Geometry check sheet. Reference: the model listing, model coordinates, mm. A direction names the side the tool comes from. Coordinates: 2 decimals unless noted, no trailing zeros. Write each loop counter-clockwise with the first axis right and the second up, starting at its lowest first coordinate (ties: lowest second). Pieces come first, ordered by that corner, then holes. Notation, with made-up numbers: (34.25, 33.5) -> (44.25, 33.5) arc R14 cw to (44.25, 57.5) -> close; hole circle Ø4 at (7, 25). An arc over 180 degrees is marked (long way). Put each result on its own line as item: value. Start each with the question number.
Autodesk Inventor part; units mm, degrees
ref_plane "YZ Plane" through (0, 0, 0) normal (1, 0, 0) x (0, 1, 0)
ref_plane "XZ Plane" through (0, 0, 0) normal (0, 1, 0) x (-1, 0, 0)
ref_plane "XY Plane" through (0, 0, 0) normal (0, 0, 1) x (1, 0, 0)
sketch "Sketch1" plane through (0, 0, 0) normal (0, 0, 1) x (1, 0, 0)
  line L0 (0, 0) -> (34, 0)
  line L1 (34, 0) -> (34, 69.8)
  line L2 (34, 69.8) -> (0, 69.8)
  line L3 (0, 69.8) -> (0, 0)
  line L4 (34, 69.8) -> (0, 69.8)
  line L5 (0, 69.8) -> (0, 0)
  line L6 (0, 0) -> (34, 0)
  line L7 (34, 0) -> (34, 69.8)
  dimension "d4" = 34
  dimension "d5" = 69.8
extrude "Extrusion1" add sketch "Sketch1" along normal blind 3.8
sketch "Sketch3" plane through (0, 0, 3.8) normal (0, 0, 1) x (1, 0, 0)
  line L0 (34, 69.8) -> (0, 69.8)
  line L1 (0, 0) -> (34, 0)
  line L2 (30, 69.8) -> (4, 69.8)
  line L3 (4, 69.8) -> (4, 0)
  line L4 (4, 0) -> (30, 0)
  line L5 (30, 0) -> (30, 69.8)
  line L6 (0, 69.8) -> (0, 0)
  line L7 (34, 0) -> (34, 69.8)
  dimension "d6" = 26
  dimension "d7" = 4
  dimension "d8" = 4
extrude "Extrusion3" add sketch "Sketch3" along normal blind 2.4 contours L5 L1 L3 L0
sketch "Sketch4" plane through (0, 0, 6.2) normal (0, 0, 1) x (1, 0, 0)
  point P0 (0, 0)
sketch "Sketch5" plane through (0, 0, 6.2) normal (0, 0, 1) x (1, 0, 0)
  line L0 (30, 69.8) -> (4, 69.8)
  line L1 (23.4, 69.8) -> (11.4, 69.8)
  line L2 (11.4, 69.8) -> (11.4, 61)
  line L3 (11.4, 61) -> (23.4, 61)
  line L4 (23.4, 61) -> (23.4, 69.8)
  point P0 (0, 0)
  dimension "d11" = 12
extrude "Extrusion4" cut sketch "Sketch5" against normal blind 8
fillet "Fillet1" radius 2 1 edges at (17, 0, 6.2)
fillet "Fillet2" radius 5 2 edges at (11.4, 65.4, 6.2) (23.4, 65.4, 6.2)
chamfer "Chamfer1" distance 2 angle 45 1 edges at (17.4, 61, 6.2)
sketch "Sketch6" plane through (0, 0, 0) normal (0, 0, -1) x (-1, 0, 0)
  line L0 (-30, 2) -> (-4, 2)
  line L1 (-30, 2) -> (-30, 69.8)
  line L2 (-4, 2) -> (-30, 2)
  line L3 (-30, 2) -> (-30, 67)
  line L4 (-30, 67) -> (-4, 67)
  line L5 (-4, 67) -> (-4, 2)
  point P0 (0, 0)
extrude "Extrusion5" cut sketch "Sketch6" against normal blind 2
properties part number "battery_cover"
Item 1: Section check D-D, the plane x = 2. Enter the section's corners in (y, z), and give its area (3 significant figures).
Item 2: Go/stop test with flat-tipped pins: P1, Ø1.9, axis at y = 36.5, z = 5, coming from the +X side; P2, Ø10, axis at x = 21.5, y = 55.5, coming from the -Z side; P3, Ø0.6, axis at x = 12, z = 0.5, coming from the +Y side. Record where each tip stops, or that it passes through.
Item 3: Section check C-C, the plane x = 26.5. Enter the section's corners in (y, z), and give its area (3 significant figures).
Item 4: Mould release check, pull along X, two halves, no side actions. Record for faces 1 (the flat face through (34, 34, 2)), 2 (the flat face through (0, 35, 2)), 3 (the flat face through (17.6, 60, 5.2)), 4 (the cylindrical face through (9.313, 65.524, 5.264)): released by +X, released by -X, zero draft, split by the parting line, or undercut.
Item 5: Section check B-B, the plane x = 12.5. Enter the section's corners in (y, z), and give its area (3 significant figures).
Item 6: Access from +Z, -Z, +X, -X, +Y, -Y to the whole of each face (thin tool, end or side, straight path). Record for faces 5 (the flat face through (4, 35, 5)), 6 (the flat face through (27, 67, 1)), 7 (the flat face through (32, 35, 3.8)), 8 (the cylindrical face through (25.487, 65.676, 5.264)).
Item 7: Scan lines: line 1 along Y through (x, z) = (28.5, 0.5); line 2 along Y through (x, z) = (14.5, 3); line 3 along Z through (x, y) = (21.5, 48). Record each from-to range of solid material in increasing order. Write a range as [from, to].
Item 8: Section check A-A, the plane y = 30.5. Enter the section's corners in (x, z), and give its area (3 significant figures).
From the geometry:
1. outline: (0, 0) -> (69.8, 0) -> (69.8, 3.8) -> (0, 3.8) -> close
1. area: 265 mm²
2. P1: x = 30
2. P2: z = 2
2. P3: y = 2
3. outline: (0, 0) -> (2, 0) -> (2, 2) -> (67, 2) -> (67, 0) -> (69.8, 0) -> (69.8, 5.82) -> (59.38, 5.82) -> (59, 6.2) -> (2, 6.2) arc R2 ccw to (0, 4.2) -> close
3. area: 298 mm²
4. face 1: released by +X
4. face 2: released by -X
4. face 3: undercut
4. face 4: undercut
5. outline: (0, 0) -> (2, 0) -> (2, 2) -> (61, 2) -> (61, 4.2) -> (59, 6.2) -> (2, 6.2) arc R2 ccw to (0, 4.2) -> close
5. area: 257 mm²
6. face 5: +Z, -X, +Y, -Y
6. face 6: -Z
6. face 7: +Z, +X, +Y, -Y
6. face 8: +Z, +Y
7. line 1: [0, 2], [67, 69.8]
7. line 2: [0, 61]
7. line 3: [2, 6.2]
8. outline: (0, 0) -> (4, 0) -> (4, 2) -> (30, 2) -> (30, 0) -> (34, 0) -> (34, 3.8) -> (30, 3.8) -> (30, 6.2) -> (4, 6.2) -> (4, 3.8) -> (0, 3.8) -> close
8. area: 140 mm²
